```python
from build123d import *

# Parameters (mm, degrees)
SKETCH2_R           = 63.5
BOSS_EXTRUDE1_DEPTH = 15
FILLET2_R           = 0.5
CUT_EXTRUDE3_REACH  = 93.047
CUT_EXTRUDE4_REACH  = 93.047
SKETCH6_R           = 2
FILLET3_R           = 5
SKETCH6_4_R         = 2
SKETCH6_4_R_2       = 4
CUT_EXTRUDE5_DEPTH  = 92.046691318


with BuildPart() as part:
    # Sketch2 → Boss-Extrude1 (new body)
    with BuildSketch(Plane(origin=(0, 0, 0), x_dir=(1, 0, 0), z_dir=(0, 1, 0))):
        with Locations(Location((0, 0, 0), (0, 0, 270))):
            Circle(SKETCH2_R)
    extrude(amount=BOSS_EXTRUDE1_DEPTH)

    # Fillet2
    fillet2_edges = [part.edges().sort_by_distance(p)[0] for p in [
        (0, 0, -63.5),
        (0, 15, -63.5),
    ]]
    fillet(fillet2_edges, radius=FILLET2_R)

    # Sketch5 → Cut-Extrude3 (cut, up to next)
    with BuildSketch(Plane.XZ, mode=Mode.PRIVATE) as cut_extrude3_sk1:
        with BuildLine():
            ThreePointArc((-4, 15.491933385), (-9.404564037, 12.94427191), (-13.497636218, 8.591496757))
            Line((-13.497636218, 8.591496757), (-39.959612231, 17.189513965))
            ThreePointArc((-39.959612231, 17.189513965), (-25.568658475, 35.192239255), (-4, 43.315701541))
            Line((-4, 43.315701541), (-4, 15.491933385))
        make_face()
    cut_extrude3_tool1 = extrude(cut_extrude3_sk1.sketch, amount=-CUT_EXTRUDE3_REACH, mode=Mode.PRIVATE) & part.part
    # Sketch5 → Cut-Extrude3 (cut, up to next)
    with BuildSketch(Plane.XZ, mode=Mode.PRIVATE) as cut_extrude3_sk2:
        with BuildLine():
            ThreePointArc((13.497636218, 8.591496757), (9.404564037, 12.94427191), (4, 15.491933385))
            Line((4, 15.491933385), (4, 43.315701541))
            ThreePointArc((4, 43.315701541), (25.568658475, 35.192239255), (39.959612231, 17.189513965))
            Line((39.959612231, 17.189513965), (13.497636218, 8.591496757))
        make_face()
    cut_extrude3_tool2 = extrude(cut_extrude3_sk2.sketch, amount=-CUT_EXTRUDE3_REACH, mode=Mode.PRIVATE) & part.part
    # Sketch5 → Cut-Extrude3 (cut, up to next)
    with BuildSketch(Plane.XZ, mode=Mode.PRIVATE) as cut_extrude3_sk3:
        with BuildLine():
            ThreePointArc((12.341997951, -10.182096375), (15.216904261, -4.94427191), (15.969772173, 0.983044626))
            Line((15.969772173, 0.983044626), (42.431748186, 9.581061834))
            ThreePointArc((42.431748186, 9.581061834), (41.370958459, -13.442239255), (28.696398536, -32.691997661))
            Line((28.696398536, -32.691997661), (12.341997951, -10.182096375))
        make_face()
    cut_extrude3_tool3 = extrude(cut_extrude3_sk3.sketch, amount=-CUT_EXTRUDE3_REACH, mode=Mode.PRIVATE) & part.part
    # Sketch5 → Cut-Extrude3 (cut, up to next)
    with BuildSketch(Plane.XZ, mode=Mode.PRIVATE) as cut_extrude3_sk4:
        with BuildLine():
            ThreePointArc((-5.869861996, -14.884378393), (0, -16), (5.869861996, -14.884378393))
            Line((5.869861996, -14.884378393), (22.224262581, -37.394279679))
            ThreePointArc((22.224262581, -37.394279679), (0, -43.5), (-22.224262581, -37.394279679))
            Line((-22.224262581, -37.394279679), (-5.869861996, -14.884378393))
        make_face()
    cut_extrude3_tool4 = extrude(cut_extrude3_sk4.sketch, amount=-CUT_EXTRUDE3_REACH, mode=Mode.PRIVATE) & part.part
    # Sketch5 → Cut-Extrude3 (cut, up to next)
    with BuildSketch(Plane.XZ, mode=Mode.PRIVATE) as cut_extrude3_sk5:
        with BuildLine():
            ThreePointArc((-15.969772173, 0.983044626), (-15.216904261, -4.94427191), (-12.341997951, -10.182096375))
            Line((-12.341997951, -10.182096375), (-28.696398536, -32.691997661))
            ThreePointArc((-28.696398536, -32.691997661), (-41.370958459, -13.442239255), (-42.431748186, 9.581061834))
            Line((-42.431748186, 9.581061834), (-15.969772173, 0.983044626))
        make_face()
    cut_extrude3_tool5 = extrude(cut_extrude3_sk5.sketch, amount=-CUT_EXTRUDE3_REACH, mode=Mode.PRIVATE) & part.part
    add(cut_extrude3_tool1.solids().sort_by_distance((-18.272678, 0, 25.150183))[0], mode=Mode.SUBTRACT)
    add(cut_extrude3_tool2.solids().sort_by_distance((18.272678, 0, 25.150183))[0], mode=Mode.SUBTRACT)
    add(cut_extrude3_tool3.solids().sort_by_distance((29.565814, 0, -9.606515))[0], mode=Mode.SUBTRACT)
    add(cut_extrude3_tool4.solids().sort_by_distance((0, 0, -31.087336))[0], mode=Mode.SUBTRACT)
    add(cut_extrude3_tool5.solids().sort_by_distance((-29.565814, 0, -9.606515))[0], mode=Mode.SUBTRACT)

    # Sketch6 → Cut-Extrude4 (cut, up to next)
    with BuildSketch(Plane.XZ, mode=Mode.PRIVATE) as cut_extrude4_sk1:
        with Locations(Location((12, 0, 0), (0, 0, 270))):
            Circle(SKETCH6_R)
    cut_extrude4_tool1 = extrude(cut_extrude4_sk1.sketch, amount=-CUT_EXTRUDE4_REACH, mode=Mode.PRIVATE) & part.part
    # Sketch6 → Cut-Extrude4 (cut, up to next)
    with BuildSketch(Plane.XZ, mode=Mode.PRIVATE) as cut_extrude4_sk2:
        with Locations(Location((0, -12, 0), (0, 0, 270))):
            Circle(SKETCH6_R)
    cut_extrude4_tool2 = extrude(cut_extrude4_sk2.sketch, amount=-CUT_EXTRUDE4_REACH, mode=Mode.PRIVATE) & part.part
    # Sketch6 → Cut-Extrude4 (cut, up to next)
    with BuildSketch(Plane.XZ, mode=Mode.PRIVATE) as cut_extrude4_sk3:
        with Locations(Location((-12, 0, 0), (0, 0, 270))):
            Circle(SKETCH6_R)
    cut_extrude4_tool3 = extrude(cut_extrude4_sk3.sketch, amount=-CUT_EXTRUDE4_REACH, mode=Mode.PRIVATE) & part.part
    # Sketch6 → Cut-Extrude4 (cut, up to next)
    with BuildSketch(Plane.XZ, mode=Mode.PRIVATE) as cut_extrude4_sk4:
        with Locations(Location((0, 12, 0), (0, 0, 270))):
            Circle(SKETCH6_R)
    cut_extrude4_tool4 = extrude(cut_extrude4_sk4.sketch, amount=-CUT_EXTRUDE4_REACH, mode=Mode.PRIVATE) & part.part
    add(cut_extrude4_tool1.solids().sort_by_distance((12, 0, 0))[0], mode=Mode.SUBTRACT)
    add(cut_extrude4_tool2.solids().sort_by_distance((0, 0, -12))[0], mode=Mode.SUBTRACT)
    add(cut_extrude4_tool3.solids().sort_by_distance((-12, 0, 0))[0], mode=Mode.SUBTRACT)
    add(cut_extrude4_tool4.solids().sort_by_distance((0, 0, 12))[0], mode=Mode.SUBTRACT)

    # Fillet3
    fillet3_edges = [part.edges().sort_by_distance(p)[0] for p in [
        (12.341997951, 7.5, -10.182096375),
        (15.969772173, 7.5, 0.983044626),
        (42.431748186, 7.5, 9.581061834),
        (28.696398536, 7.5, -32.691997661),
        (13.497636218, 7.5, 8.591496757),
        (4, 7.5, 15.491933385),
        (4, 7.5, 43.315701541),
        (39.959612231, 7.5, 17.189513965),
        (-15.969772173, 7.5, 0.983044626),
        (-12.341997951, 7.5, -10.182096375),
        (-28.696398536, 7.5, -32.691997661),
        (-42.431748186, 7.5, 9.581061834),
        (-5.869861996, 7.5, -14.884378393),
        (5.869861996, 7.5, -14.884378393),
        (22.224262581, 7.5, -37.394279679),
        (-22.224262581, 7.5, -37.394279679),
        (-4, 7.5, 15.491933385),
        (-13.497636218, 7.5, 8.591496757),
        (-39.959612231, 7.5, 17.189513965),
        (-4, 7.5, 43.315701541),
    ]]
    fillet(fillet3_edges, radius=FILLET3_R)

    # Sketch6_4 → Cut-Extrude5 (cut, through all)
    with BuildSketch(Plane.XZ):
        with Locations(Location((12, 0, 0), (0, 0, 270))):
            Circle(SKETCH6_4_R)
        with Locations(Location((0, -12, 0), (0, 0, 270))):
            Circle(SKETCH6_4_R)
        with Locations(Location((-12, 0, 0), (0, 0, 270))):
            Circle(SKETCH6_4_R)
        with Locations(Location((0, 12, 0), (0, 0, 270))):
            Circle(SKETCH6_4_R)
        with Locations(Location((0, 0, 0), (0, 0, 270))):
            Circle(SKETCH6_4_R_2)
    extrude(amount=-CUT_EXTRUDE5_DEPTH, mode=Mode.SUBTRACT)


solid = part.part
```
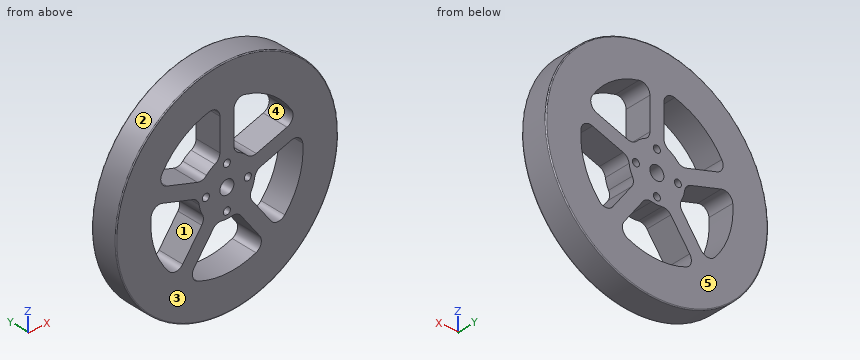
Part model, mm, in its own coordinate system. Face numbers are marked on the shaded views. A direction names the side the tool comes from. Coordinates: 2 decimals unless noted, no trailing zeros. Write each loop counter-clockwise with the first axis right and the second up, starting at its lowest first coordinate (ties: lowest second). Pieces come first, ordered by that corner, then holes.
Item 1: Slice it at B-B (y = 2.75). Count the separate pieces of the cut face and the enclosed holes in it, and give its area (3 significant figures).
Item 2: Probe line 1 (X direction, y = 5, z = 0); line 2 (Z direction, x = 25, y = 10.25); line 3 (X direction, y = 3.75, z = -17.5). List the from-to ranges inside material, lowest first.
Item 3: Mould opens along Z. For the marked faces 1, 2 and 3 say: released by +Z, released by -Z, zero draft, split by the parting line, or undercut.
Item 4: Pin check, flat tips, straight feed: pin 1 (4.5 mm diameter, centred on y = 6, z = 28, fed in from -X); pin 2 (4 mm diameter, centred on y = 6.5, z = 15.5, fed in from +X); pin 3 (2 mm diameter, centred on y = 12, z = -20, fed in from -X). Stop position of each tip, or through.
Item 5: Which spindle directions (+Z, -Z, +X, -X, +Y, -Y) get a long thin tool onto all of the face, cutting with end or side? Do the marked faces 4 and 5. Say none if no direction does.
Item 6: Slice it at A-A (x = 0). Write the cut outline in (y, z), and give its area (3 significant figures).
Results found:
1. separate pieces: 1
1. enclosed holes: 10
1. area: 8,630 mm2
2. line 1: x = -63.5 to -43.5, -16.62 to -14, -10 to -4, 4 to 10, 14 to 16.62, 43.5 to 63.5
2. line 2: z = -58.37 to -27.6, 3.92 to 12.33, 35.6 to 58.37
2. line 3: x = -61.04 to -39.82, -17.66 to -7.76, 7.76 to 17.66, 39.82 to 61.04
3. face 1: undercut
3. face 2: split by the parting line
3. face 3: zero draft
4. pin 1: stops at x = -58.04
4. pin 2: stops at x = 62.05
4. pin 3: stops at x = -60.59
5. face 4: +Y, -Y
5. face 5: +Z, -Z, +X, -X, +Y
6. outline: (0, -63) arc R0.5 ccw to (0.5, -63.5) - (14.5, -63.5) arc R0.5 ccw to (15, -63) - (15, -43.5) - (0, -43.5) - close; (0, -16) - (15, -16) - (15, -14) - (0, -14) - close; (0, -10) - (15, -10) - (15, -4) - (0, -4) - close; (0, 4) - (15, 4) - (15, 10) - (0, 10) - close; (0, 14) - (15, 14) - (15, 63) arc R0.5 ccw to (14.5, 63.5) - (0.5, 63.5) arc R0.5 ccw to (0, 63) - close
6. area: 1,250 mm2
